from build123d import *

# Parameters (mm, degrees)
MOTOR_DEPTH           = 15
GEARBOX_DEPTH         = 9
CUT_EXTRUDE1_START    = 0.8
SKETCH6_OUTSIDE_W     = 19.728
SKETCH6_OUTSIDE_H     = 17.728
CUT_EXTRUDE1_DEPTH    = 2.3
SKETCH5_R             = 2
GEARBOX_BEARING_DEPTH = 1
SHAFT_START           = 1
SHAFT_DEPTH           = 9
ENCODER_BASE_START    = -6.1
ENCODER_BASE_DEPTH    = 6.1
SKETCH7_OUTSIDE_W     = 23.112
SKETCH7_OUTSIDE_H     = 29.112
SKETCH7_OUTSIDE_R     = 4.55
SKETCH7_OUTSIDE_W_2   = 10.4
SKETCH7_OUTSIDE_H_2   = 4.6
CUT_EXTRUDE3_DEPTH    = 4.9
SKETCH8_W             = 9.6
SKETCH8_H             = 4.1
CUT_EXTRUDE4_DEPTH    = 3.84


with BuildPart() as part:
    # Sketch1 → motor (new body)
    with BuildSketch(Plane.XY):
        with BuildLine():
            Line((-3.62, 5), (3.62, 5))
            ThreePointArc((3.62, 5), (6, 0), (3.62, -5))
            Line((3.62, -5), (-3.62, -5))
            ThreePointArc((-3.62, -5), (-6, 0), (-3.62, 5))
        make_face()
    extrude(amount=MOTOR_DEPTH)

    # Sketch3 → gearbox (add)
    with BuildSketch(Plane.XY.offset(15)):
        with BuildLine():
            Line((-5, -5), (5, -5))
            ThreePointArc((5, -5), (5.707106781, -4.707106781), (6, -4))
            Line((6, -4), (6, 4))
            ThreePointArc((6, 4), (5.707106781, 4.707106781), (5, 5))
            Line((5, 5), (-5, 5))
            ThreePointArc((-5, 5), (-5.707106781, 4.707106781), (-6, 4))
            Line((-6, 4), (-6, -4))
            ThreePointArc((-6, -4), (-5.707106781, -4.707106781), (-5, -5))
        make_face()
    extrude(amount=GEARBOX_DEPTH)

    # Sketch6 outside → Cut-Extrude1 (cut)
    with BuildSketch(Plane.XY.offset(15).offset(CUT_EXTRUDE1_START)):
        Rectangle(SKETCH6_OUTSIDE_W, SKETCH6_OUTSIDE_H)
        with BuildLine():
            Line((-4, 4.5), (4, 4.5))
            ThreePointArc((4, 4.5), (5.060660172, 4.060660172), (5.5, 3))
            Line((5.5, 3), (5.5, -3))
            ThreePointArc((5.5, -3), (5.060660172, -4.060660172), (4, -4.5))
            Line((4, -4.5), (-4, -4.5))
            ThreePointArc((-4, -4.5), (-5.060660172, -4.060660172), (-5.5, -3))
            Line((-5.5, -3), (-5.5, 3))
            ThreePointArc((-5.5, 3), (-5.060660172, 4.060660172), (-4, 4.5))
        make_face(mode=Mode.SUBTRACT)
    extrude(amount=CUT_EXTRUDE1_DEPTH, mode=Mode.SUBTRACT)

    # Sketch5 → gearbox-bearing (add)
    with BuildSketch(Plane.XY.offset(24)):
        Circle(SKETCH5_R)
    extrude(amount=GEARBOX_BEARING_DEPTH)

    # Sketch4 → shaft (add)
    with BuildSketch(Plane.XY.offset(24).offset(SHAFT_START)):
        with BuildLine():
            Line((-1.118033989, 1), (1.118033989, 1))
            ThreePointArc((1.118033989, 1), (0, -1.5), (-1.118033989, 1))
        make_face()
    extrude(amount=SHAFT_DEPTH)

    # Sketch2 → encoder-base (add)
    with BuildSketch(Plane.XY.offset(ENCODER_BASE_START)):
        with BuildLine():
            Line((6, 0), (6, -13))
            Line((6, -13), (-6, -13))
            Line((-6, -13), (-6, 0))
            ThreePointArc((-6, 0), (-5.37464767, 2.768772291), (-3.62, 5))
            Line((-3.62, 5), (3.62, 5))
            ThreePointArc((3.62, 5), (5.37464767, 2.768772291), (6, 0))
        make_face()
    extrude(amount=ENCODER_BASE_DEPTH)

    # Sketch7 outside → Cut-Extrude3 (cut)
    with BuildSketch(Plane(origin=(0, 0, -6.1), x_dir=(-1, 0, 0), z_dir=(0, 0, -1))):
        with Locations((0, -4)):
            Rectangle(SKETCH7_OUTSIDE_W, SKETCH7_OUTSIDE_H)
        Circle(SKETCH7_OUTSIDE_R, mode=Mode.SUBTRACT)
        Polygon((4.939339828, -2.110912703), (2.110912703, -4.939339828), (3.171572875, -6), (6, -3.171572875), align=None, mode=Mode.SUBTRACT)
        Polygon((-2.110912703, -4.939339828), (-3.171572875, -6), (-6, -3.171572875), (-4.939339828, -2.110912703), align=None, mode=Mode.SUBTRACT)
        with Locations((0, -10.7)):
            Rectangle(SKETCH7_OUTSIDE_W_2, SKETCH7_OUTSIDE_H_2, mode=Mode.SUBTRACT)
    extrude(amount=-CUT_EXTRUDE3_DEPTH, mode=Mode.SUBTRACT)

    # Sketch8 → Cut-Extrude4 (cut)
    with BuildSketch(Plane.XZ.offset(13)):
        with Locations((0, -3.65)):
            Rectangle(SKETCH8_W, SKETCH8_H)
    extrude(amount=-CUT_EXTRUDE4_DEPTH, mode=Mode.SUBTRACT)


solid = part.part
Build history of the part. All positions in model axes, mm. A direction names the side the tool comes from. Round coordinates to 2 decimals unless told otherwise and drop trailing zeros. Order: outer loops, then holes, each group sorted by start corner. A loop starts at its lowest first (then second) coordinate and runs counter-clockwise, first axis right, second up. Notation, with made-up numbers: M 13,-23.5 L 39,-23.5 A17 ccw 39,-8.5 Z; hole C 7,68.25 d6. An arc over 180 degrees is marked long. Use CSV: the item, a comma, the result in double quotes. Start each with the question number.
(1) Drill centre lines: probe 1 along Z at (x, y) = (-2.25, -0.25); probe 2 along Z at (x, y) = (4.75, -12); probe 3 along Y at (x, z) = (1.75, 5.5). Where is each one in solid material? Low to high.
(2) Tool access for faces 4 (the face through (0, 4.5, 17)), 5 (the face through (0, -4.5, 17)), 6 (the face through (-5, -4, 15)), 7 (the face through (0, 1.4, 25)), 8 (the face through (-4.566, -4.606, -3.684)): list every direction of +Z, -Z, +X, -X, +Y, -Y with a clear straight run to the whole face (end or side of a thin tool).
(3) Cut at C-C on z = -0.5. List the corners of the cut face in (x, y).
(4) Cut at D-D on z = 11. List the corners of the cut face in (x, y).
(5) Flat gauge pins, fed straight in: P1, Ø6, axis at x = -1.5, y = -9.5, coming from the +Z side; P2, Ø2.5, axis at x = 0.5, z = 28, coming from the +Y side; P3, Ø0.7, axis at x = 0, z = 17, coming from the +Y side. Where does each tip first touch, or does it go through?
(6) Cut at B-B on z = 20.5. List the corners of the cut face in (x, y).
(7) Mould opens along Y. For faces 1 (the face through (4.8, -11, -4)), 2 (the face through (5.715, 4.699, 21.009)), 3 (the face through (0, -6, -1.2)) say: +Y half, -Y half, draft (parallel to the pull), parting line (faces both ways), or undercut.
Findings:
1,probe 1,"z = -6.1 to 24"
1,probe 2,"z = -6.1 to -5.7, -1.6 to 0"
1,probe 3,"y = -5 to 5"
2,face 4,"+X, -X, +Y"
2,face 5,"+X, -X, -Y"
2,face 6,"-X, -Y"
2,face 7,"+Z"
2,face 8,"-Z, -X"
3,outline,"M -6,-13 L 6,-13 L 6,0 A6.44 ccw 3.62,5 L -3.62,5 A6.44 ccw -6,0 Z"
4,outline,"M -3.62,-5 L 3.62,-5 A6.44 ccw 3.62,5 L -3.62,5 A6.44 ccw Z"
5,P1,"stops at z = 0"
5,P2,"stops at y = 1"
5,P3,"stops at y = 4.5"
6,outline,"M -6,-4 A1 ccw -5,-5 L 5,-5 A1 ccw 6,-4 L 6,4 A1 ccw 5,5 L -5,5 A1 ccw -6,4 Z"
7,face 1,"draft"
7,face 2,"+Y half"
7,face 3,"undercut"
